from build123d import *

# Parameters (mm, degrees)
BOSS_EXTRUDE1_DEPTH = 6.33
SKETCH2_R           = 2.15
CUT_EXTRUDE1_DEPTH  = 11.529667611


with BuildPart() as part:
    # Sketch1 → Boss-Extrude1 (new body)
    with BuildSketch(Plane(origin=(0, 0, 0), x_dir=(1, 0, 0), z_dir=(0, 1, 0))):
        with BuildLine():
            Line((-5.95, -5.95), (5.95, -5.95))
            ThreePointArc((5.95, -5.95), (4.046256646, 0), (5.95, 5.95))
            Line((5.95, 5.95), (-5.95, 5.95))
            ThreePointArc((-5.95, 5.95), (-4.046256646, 0), (-5.95, -5.95))
        make_face()
    extrude(amount=-BOSS_EXTRUDE1_DEPTH)

    # Sketch2 → Cut-Extrude1 (cut, through all)
    with BuildSketch(Plane(origin=(0, 0, 0), x_dir=(1, 0, 0), z_dir=(0, 1, 0))):
        with Locations(Location((0, 0, 0), (0, 0, 270))):
            Circle(SKETCH2_R)
    extrude(amount=-CUT_EXTRUDE1_DEPTH, mode=Mode.SUBTRACT)


solid = part.part
Read the model definition and answer for the solid it produces. Units are mm, in the model's axes. Coordinates: 2 decimals unless noted, no trailing zeros. Loops run counter-clockwise (first coordinate to the right, second up) from the corner with the lowest first, then second, coordinate; pieces in that order, holes last. Notation, with made-up numbers: (36, 10) -> (89, 10) arc R31 ccw to (89, 41) -> close; hole circle Ø4 at (-3, -20). An arc over 180 degrees is marked (long way). Answer in a Markdown table with one row per item.
Item 1: A cutting plane is placed at A-A on z = 0. Determine the outline of the cut face in (x, y).
Returned:
| item | result |
|---|---|
| outline | (-4.05, -6.33) -> (-2.15, -6.33) -> (-2.15, 0) -> (-4.05, 0) -> close; (2.15, -6.33) -> (4.05, -6.33) -> (4.05, 0) -> (2.15, 0) -> close |
Item 2: A cutting plane is placed at B-B on x = 0. Determine the outline of the cut face in (y, z).
Returned:
| item | result |
|---|---|
| outline | (-6.33, -5.95) -> (0, -5.95) -> (0, -2.15) -> (-6.33, -2.15) -> close; (-6.33, 2.15) -> (0, 2.15) -> (0, 5.95) -> (-6.33, 5.95) -> close |
Item 3: Straight lines are drawn through the part: line 1 along Z through (x, y) = (5.5, -1.75); line 2 along X through (y, z) = (-2.25, -0.75); line 3 along Z through (x, y) = (-1.5, -4.5). For each, find the intervals that lie inside material, in ascending order. Write a range as [from, to].
Returned:
| item | result |
|---|---|
| line 1 | z = [-5.95, -5.26], [5.26, 5.95] |
| line 2 | x = [-4.07, -2.01], [2.01, 4.07] |
| line 3 | z = [-5.95, -1.54], [1.54, 5.95] |
Item 4: A cutting plane is placed at D-D on z = 2.5. Determine the outline of the cut face in (x, y), plus the area to 3 significant figures.
Returned:
| item | result |
|---|---|
| outline | (-4.36, -6.33) -> (4.36, -6.33) -> (4.36, 0) -> (-4.36, 0) -> close |
| area | 55.1 mm^2 |
Item 5: Each of these flat-tipped pins is pushed along its axis until it touches: P1, Ø2, axis at y = -4, z = -2, coming from the +X side; P2, Ø1.5, axis at y = -3, z = 1.5, coming from the +X side; P3, Ø2, axis at y = -1, z = -4.5, coming from the -X side. Where does it stop, or does it pass through?
Returned:
| item | result |
|---|---|
| P1 | stops at x = 4.5 |
| P2 | stops at x = 4.3 |
| P3 | stops at x = -5.65 |
Item 6: A cutting plane is placed at C-C on y = -6. Determine the outline of the cut face in (x, z), plus the area to 3 significant figures.
Returned:
| item | result |
|---|---|
| outline | (-5.95, -5.95) -> (5.95, -5.95) arc R10.25 cw to (5.95, 5.95) -> (-5.95, 5.95) arc R10.25 cw to start; hole circle Ø4.3 at (0, 0) |
| area | 96.3 mm^2 |
